```python
from build123d import *

# Parameters (mm, degrees)
BASEHEAD_DEPTH = 5.675
SKETCH4_W      = 0.6
SKETCH4_H      = 11.005553499


with BuildPart() as part:
    # Sketch1 → BaseHead (new body)
    with BuildSketch(Plane(origin=(0, 0, 0), x_dir=(0, 0, -1), z_dir=(1, 0, 0))):
        Polygon((6.5, 3.75277675), (6.5, -3.75277675), (0, -7.505553499), (-6.5, -3.75277675), (-6.5, 3.75277675), (0, 7.505553499), align=None)
    extrude(amount=BASEHEAD_DEPTH)

    # BodySke → BaseBody (revolve)
    with BuildSketch(Plane.XY, mode=Mode.PRIVATE) as basebody_sk:
        Polygon((0, 0), (30.675, 0), (30.675, 3.3095), (29.9845, 4), (0, 4), align=None)
    revolve(basebody_sk.sketch.rotate(Axis((0, 0, 0), (1, 0, 0)), 90), axis=Axis((0, 0, 0), (1, 0, 0)))

    # Sketch3 → HeadChamfer (revolve, cut)
    with BuildSketch(Plane.XY):
        Polygon((0, 6.5), (3.46730793, 12.505553499), (3.46730793, 17.505553499), (-10, 17.505553499), (-10, 6.5), align=None)
    revolve(axis=Axis((0, 0, 0), (1, 0, 0)), mode=Mode.SUBTRACT)

    # Sketch4 → BearingFace (revolve, cut)
    with BuildSketch(Plane.XY, mode=Mode.PRIVATE) as bearingface_sk:
        with Locations((5.375, 12.00277675)):
            Rectangle(SKETCH4_W, SKETCH4_H)
    revolve(bearingface_sk.sketch.rotate(Axis((0, 0, 0), (1, 0, 0)), 270), axis=Axis((0, 0, 0), (1, 0, 0)), mode=Mode.SUBTRACT)


solid = part.part
```
Here's how the part is built. I have some questions about the finished solid (model axes, mm). A direction names the side the tool comes from. Coordinates: 2 decimals unless noted, no trailing zeros. Order: outer loops, then holes, each group sorted by start corner. A loop starts at its lowest first (then second) coordinate and runs counter-clockwise, first axis right, second up.
1) Which directions (+Z, -Z, +X, -X, +Y, -Y) give clear straight access to the entire face, cutting with the end or side of a thin tool? Please do faces 1 (the face through (5.075, -3, -6)), 2 (the face through (5.075, -7, 0)), 3 (the face through (5.675, -3, -3)).
2) Will these pins go through, and if not, where does the flat tip stop? pin 1 (2 mm diameter, centred on x = 6.5, y = 5, fed in from -Z); pin 2 (8 mm diameter, centred on x = 13, y = -1.5, fed in from +Z); pin 3 (3.5 mm diameter, centred on y = 2, z = -5.5, fed in from +X) (3 decimals).
3) Imagine slicing it at B-B on x = 13. List the corners of the cut face in (y, z) for me, and give its area (3 significant figures).
4) I need wall thicknesses on line 1 (Z direction, x = 17, y = -2.25); line 2 (X direction, y = 2.5, z = -3.5) (3 decimals); line 3 (Y direction, x = 13.5, z = -2.5). Which ranges of each line are inside material? Lowest first, please.
5) Imagine slicing it at A-A on x = 3. List the corners of the cut face in (y, z) for me, and give its area (3 significant figures).
Response values:
1. face 1: -Z, +X, -Y
1. face 2: +X, -Y
1. face 3: +X
2. pin 1: stops at z = -4.75
2. pin 2: stops at z = 4
2. pin 3: stops at x = 5.675
3. outline: circle Ø8 at (0, 0)
3. area: 50.3 mm2
4. line 1: z = -3.31 to 3.31
4. line 2: x = 0 to 5.675
4. line 3: y = -3.12 to 3.12
5. outline: (-7.51, 0) - (-3.75, -6.5) - (3.75, -6.5) - (7.51, 0) - (3.75, 6.5) - (-3.75, 6.5) - close
5. area: 146 mm2
